from build123d import *

# Parameters (mm, degrees)
SKETCH1_R           = 73
SKETCH1_R_2         = 60
SKETCH1_R_3         = 3.25
BOSS_EXTRUDE1_DEPTH = 3.275


with BuildPart() as part:
    # Sketch1 → Boss-Extrude1 (new body)
    with BuildSketch(Plane(origin=(0, 0, 0), x_dir=(1, 0, 0), z_dir=(0, 1, 0))):
        Circle(SKETCH1_R)
        Circle(SKETCH1_R_2, mode=Mode.SUBTRACT)
        with Locations((-48.083261121, 48.083261121)):
            Circle(SKETCH1_R_3, mode=Mode.SUBTRACT)
        with Locations((-68, 0)):
            Circle(SKETCH1_R_3, mode=Mode.SUBTRACT)
        with Locations((0, 68)):
            Circle(SKETCH1_R_3, mode=Mode.SUBTRACT)
        with Locations((48.083261121, 48.083261121)):
            Circle(SKETCH1_R_3, mode=Mode.SUBTRACT)
        with Locations((68, 0)):
            Circle(SKETCH1_R_3, mode=Mode.SUBTRACT)
        with Locations((48.083261121, -48.083261121)):
            Circle(SKETCH1_R_3, mode=Mode.SUBTRACT)
        with Locations((0, -68)):
            Circle(SKETCH1_R_3, mode=Mode.SUBTRACT)
        with Locations((-48.083261121, -48.083261121)):
            Circle(SKETCH1_R_3, mode=Mode.SUBTRACT)
    extrude(amount=BOSS_EXTRUDE1_DEPTH)


solid = part.part
Geometry: final body of the model. Coordinates: model frame, mm. Give positions to 0.01 mm unless a question says otherwise; leave off trailing zeros. Write each loop counter-clockwise with the first axis right and the second up, starting at its lowest first coordinate (ties: lowest second). Pieces come first, ordered by that corner, then holes.
(1) Mould query, pull axis Z, two halves, no side actions, for faces 1 (the cylindrical face through (-15.825, 1.615, 71.264)), 2 (the cylindrical face through (-59.94, 1.61, -2.64)), 3 (the flat face through (-11.2, 3.275, 59.1)). Classes: released by +Z, released by -Z, zero draft, split by the parting line, or undercut.
(2) Cut plane B-B, the plane x = 0. Return loops of the section in (y, z) (3 decimals), then the cut area to 3 significant figures.
(3) Cut plane D-D, the plane z = 26. Return loops of the section in (x, y) (3 decimals).
(4) Cut plane C-C, the plane y = 1.4. Give the number of separate pieces and of enclosed holes in the cut face, then the cut area to 3 significant figures.
(5) Ray query, line 1 (X direction, y = 1.9, z = 0); line 2 (X direction, y = 1.8, z = -1); line 3 (Z direction, x = 3, y = 0.85). Return the intervals inside material, ascending.
(6) First-contact query: P1, Ø8.5, axis at x = -68, z = 0, coming from the -Y side; P2, Ø1.5, axis at x = -3.5, y = 0.5, coming from the -Z side; P3, Ø1.5, axis at y = 3, z = -40.5, coming from the +X side. Flat tips, straight axial feed; report the tip coordinate or a pass-through.
(7) Cut plane A-A, the plane z = 0. Return loops of the section in (x, y) (3 decimals), then the cut area to 3 significant figures.
Values follow:
1. face 1: split by the parting line
1. face 2: undercut
1. face 3: zero draft
2. outline: (0, -73) - (3.275, -73) - (3.275, -71.25) - (0, -71.25) - close; (0, -64.75) - (3.275, -64.75) - (3.275, -60) - (0, -60) - close; (0, 60) - (3.275, 60) - (3.275, 64.75) - (0, 64.75) - close; (0, 71.25) - (3.275, 71.25) - (3.275, 73) - (0, 73) - close
2. area: 42.6 mm2
3. outline: (-68.213, 0) - (-54.074, 0) - (-54.074, 3.275) - (-68.213, 3.275) - close; (54.074, 0) - (68.213, 0) - (68.213, 3.275) - (54.074, 3.275) - close
4. separate pieces: 1
4. enclosed holes: 9
4. area: 5,170 mm2
5. line 1: x = -73 to -71.25, -64.75 to -60, 60 to 64.75, 71.25 to 73
5. line 2: x = -72.99 to -71.09, -64.91 to -59.99, 59.99 to 64.91, 71.09 to 72.99
5. line 3: z = -72.94 to -69.25, -66.75 to -59.92, 59.92 to 66.75, 69.25 to 72.94
6. P1: stops at y = 0
6. P2: stops at z = -72.95
6. P3: stops at x = 61.23
7. outline: (-73, 0) - (-71.25, 0) - (-71.25, 3.275) - (-73, 3.275) - close; (-64.75, 0) - (-60, 0) - (-60, 3.275) - (-64.75, 3.275) - close; (60, 0) - (64.75, 0) - (64.75, 3.275) - (60, 3.275) - close; (71.25, 0) - (73, 0) - (73, 3.275) - (71.25, 3.275) - close
7. area: 42.6 mm2
